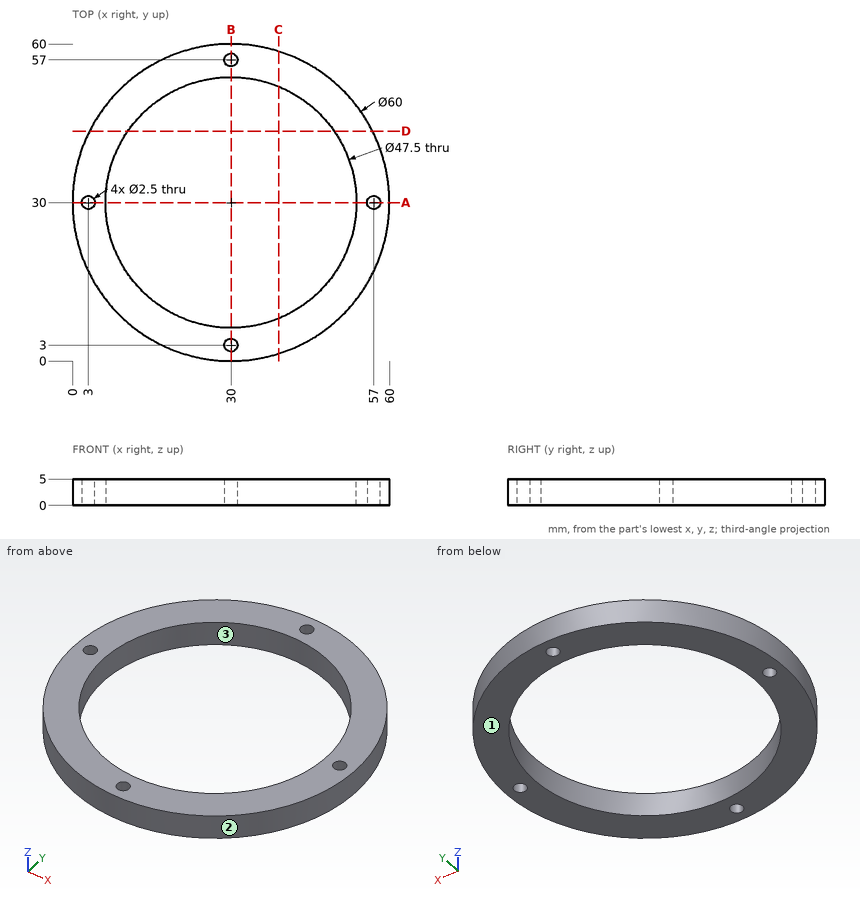
Source: three-view drawing plus pictorial views. Frame: mm from the lowest corner of the part. Give positions to 0.01 mm unless a question says otherwise; leave off trailing zeros. Loops run counter-clockwise (first coordinate to the right, second up) from the corner with the lowest first, then second, coordinate; pieces in that order, holes last. Notation, with made-up numbers: M -19.75,-3 L 35.25,-3 A15 cw 35.25,7 Z; hole C -37,18.25 d7. An arc over 180 degrees is marked long. Use CSV: the item, a comma, the result in double quotes.
(1) Pin query (flat end, axial travel): P1, Ø1.5, axis at x = 30, y = 3, coming from the -Z side; P2, Ø1.5, axis at x = 7.5, z = 2, coming from the -Y side; P3, Ø1, axis at y = 8, z = 2.5, coming from the -X side; P4, Ø2, axis at y = 31.5, z = 3, coming from the -X side. Return the tip coordinate at first contact, or that it passes through.
Outcome:
P1,"passes through"
P2,"stops at y = 9.34"
P3,"stops at x = 9.08"
P4,"stops at x = 0"
(2) Section C-C, the plane x = 39. Return loops of the section in (y, z).
Outcome:
outline,"M 1.38,0 L 8.02,0 L 8.02,5 L 1.38,5 Z; M 51.98,0 L 58.62,0 L 58.62,5 L 51.98,5 Z"
(3) Pull-direction query (X, two-part tool) for the marked faces 1, 2 and 3; classes: pulls with the +X half, pulls with the -X half, needs draft (parallel to the pull), parting line crosses it, or undercut.
Outcome:
face 1,"needs draft"
face 2,"parting line crosses it"
face 3,"undercut"
(4) Section A-A, the plane y = 30. Return loops of the section in (x, z), plus the area to 3 significant figures.
Outcome:
outline,"M 0,0 L 1.75,0 L 1.75,5 L 0,5 Z; M 4.25,0 L 6.25,0 L 6.25,5 L 4.25,5 Z; M 53.75,0 L 55.75,0 L 55.75,5 L 53.75,5 Z; M 58.25,0 L 60,0 L 60,5 L 58.25,5 Z"
area,"37.5 mm²"
(5) Section D-D, the plane y = 43.5. Return loops of the section in (x, z).
Outcome:
outline,"M 3.21,0 L 10.46,0 L 10.46,5 L 3.21,5 Z; M 49.54,0 L 56.79,0 L 56.79,5 L 49.54,5 Z"
(6) Material intervals for L1, parallel to Y at x = 30, z = 2; L2, parallel to Y at x = 29.5, z = 4.75; L3, parallel to Y at x = 57, z = 2.9, sorted ascending. Write a range as [from, to].
Outcome:
L1,"y = [0, 1.75], [4.25, 6.25], [53.75, 55.75], [58.25, 60]"
L2,"y = [0, 1.85], [4.15, 6.26], [53.74, 55.85], [58.15, 60]"
L3,"y = [16.92, 28.75], [31.25, 43.08]"
